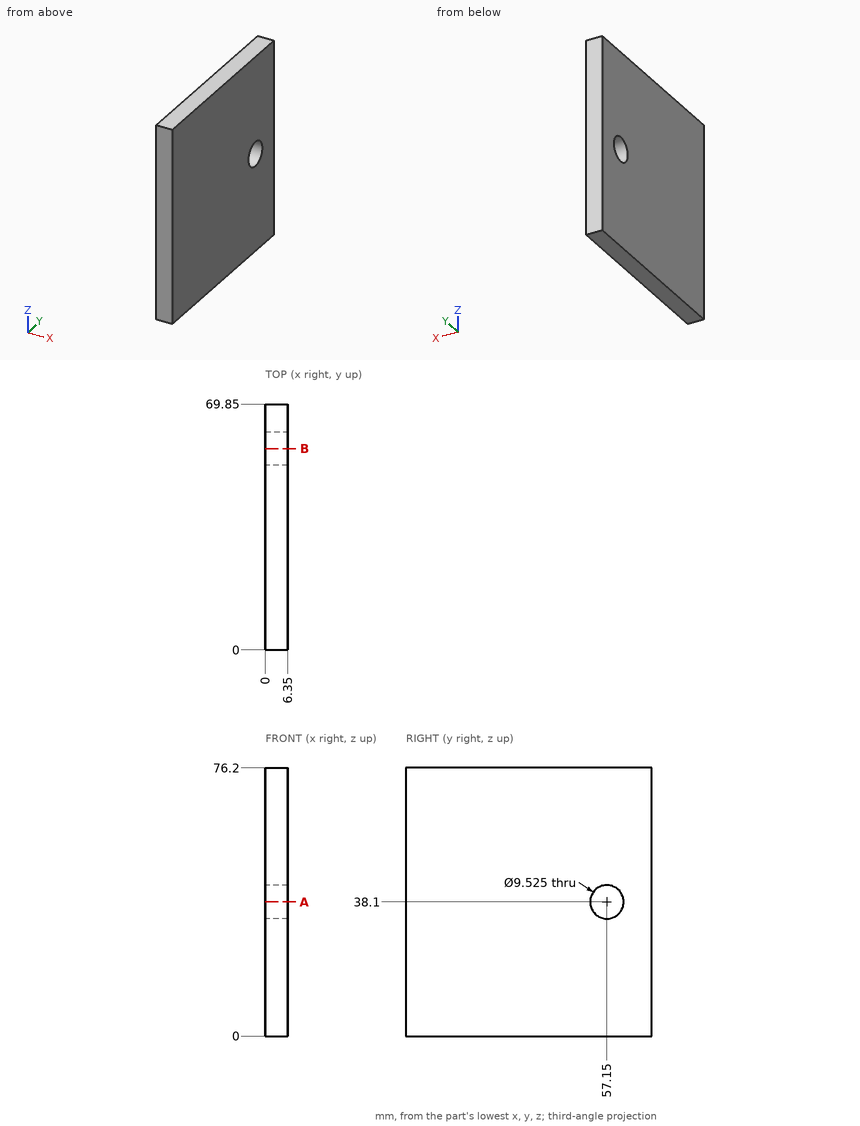
Part print with two shaded views. Sizes in mm from the minimum x, y, z corner. Coordinates: 2 decimals unless noted, no trailing zeros. Loops run counter-clockwise (first coordinate to the right, second up) from the corner with the lowest first, then second, coordinate; pieces in that order, holes last. Notation, with made-up numbers: (-25.75, -28.75) - (-10.75, -28.75) arc R20 cw to (-10.75, -2.75) - close; hole circle Ø11 at (48, 18.25). An arc over 180 degrees is marked (long way). Write each question's results on one line, items separated by ' | '. Start each with the question number.
Q1. Probe line 1 along Z through (x, y) = (4.75, 57.15); line 2 along Y through (x, z) = (5.5, 37.5); line 3 along Y through (x, z) = (5.75, 39). List the from-to ranges inside material, lowest first.
Q2. Slice it at A-A on z = 38.1. Give the cut face in (x, y), and give its area (3 significant figures).
Q3. Slice it at B-B on y = 57.15. Give the cut face in (x, z).
Answer:
1) line 1: z = 0 to 33.34, 42.86 to 76.2 | line 2: y = 0 to 52.43, 61.87 to 69.85 | line 3: y = 0 to 52.47, 61.83 to 69.85
2) outline: (0, 0) - (6.35, 0) - (6.35, 52.39) - (0, 52.39) - close; (0, 61.91) - (6.35, 61.91) - (6.35, 69.85) - (0, 69.85) - close | area: 383 mm2
3) outline: (0, 0) - (6.35, 0) - (6.35, 33.34) - (0, 33.34) - close; (0, 42.86) - (6.35, 42.86) - (6.35, 76.2) - (0, 76.2) - close
